Autodesk Inventor part; units mm, degrees
ref_plane "YZ Plane" through (0, 0, 0) normal (1, 0, 0) x (0, 1, 0)
ref_plane "XZ Plane" through (0, 0, 0) normal (0, 1, 0) x (-1, 0, 0)
ref_plane "XY Plane" through (0, 0, 0) normal (0, 0, 1) x (1, 0, 0)
sketch "Sketch6" plane through (0, 0, 0) normal (0, 1, 0) x (-1, 0, 0)
  line L0 (-10, -10) -> (10, -10)
  line L1 (10, -10) -> (10, 10)
  line L2 (10, 10) -> (-10, 10)
  line L3 (-10, 10) -> (-10, -10)
  line L4 (-10, -10) -> (10, 10) construction
  line L5 (10, -10) -> (-10, 10) construction
  point P0 (0, 0)
  dimension "d28" = 20
  dimension "d29" = 20
extrude "Extrusion6" add sketch "Sketch6" along normal blind 1
sketch "Sketch7" plane through (0, 1, 0) normal (0, 1, 0) x (1, 0, 0)
  circle A0 centre (-8.5, -8.5) radius 1
  line L0 (-10, 10) -> (-10, -10)
  line L1 (-10, -10) -> (10, -10)
  point P0 (0, 0)
  dimension "d32" = 2
  dimension "d33" = 0.5
  dimension "d34" = 0.5
extrude "Extrusion7" add sketch "Sketch7" along normal blind 10
sketch "Sketch8" plane through (0, 1, 0) normal (0, 1, 0) x (1, 0, 0)
  circle A0 centre (-8.5, 8.5) radius 1
  line L0 (-10, 10) -> (-10, -10)
  line L1 (10, 10) -> (-10, 10)
  point P0 (0, 0)
  dimension "d37" = 2
  dimension "d38" = 0.5
  dimension "d39" = 0.5
extrude "Extrusion8" add sketch "Sketch8" along normal blind 10
sketch "Sketch9" plane through (0, 1, 0) normal (0, 1, 0) x (1, 0, 0)
  circle A0 centre (8.5, -8.5) radius 1
  line L0 (10, -10) -> (10, 10)
  line L1 (-10, -10) -> (10, -10)
  point P0 (0, 0)
  dimension "d42" = 2
  dimension "d43" = 0.5
  dimension "d44" = 0.5
extrude "Extrusion9" add sketch "Sketch9" along normal blind 10
sketch "Sketch10" plane through (0, 1, 0) normal (0, 1, 0) x (1, 0, 0)
  circle A0 centre (8.5, 8.5) radius 1
  line L0 (10, -10) -> (10, 10)
  line L1 (10, 10) -> (-10, 10)
  point P0 (0, 0)
  dimension "d47" = 2
  dimension "d48" = 0.5
  dimension "d49" = 0.5
extrude "Extrusion10" add sketch "Sketch10" along normal blind 10
sketch "Sketch11" plane through (-8.5, 11, 8.5) normal (0, 1, 0) x (1, 0, 0)
  line L0 (18.75, 18.75) -> (-1.75, 18.75)
  line L1 (-1.75, 18.75) -> (-1.75, -1.75)
  line L2 (-1.75, -1.75) -> (18.75, -1.75)
  line L3 (18.75, -1.75) -> (18.75, 18.75)
  line L4 (18.75, 18.75) -> (-1.75, -1.75) construction
  line L5 (-1.75, 18.75) -> (18.75, -1.75) construction
  point P0 (8.5, 8.5)
  dimension "d52" = 20.5
  dimension "d53" = 20.5
extrude "Extrusion11" add sketch "Sketch11" along normal blind 0.5
sketch "Sketch12" plane through (-8.5, 11.5, 8.5) normal (0, 1, 0) x (1, 0, 0)
  point P0 (8.5, 8.5)
sketch "Sketch13" plane through (-8.5, 11.5, 8.5) normal (0, 1, 0) x (1, 0, 0)
  line L0 (0.75, 0.75) -> (-1.25, 0.75)
  line L1 (-1.25, 0.75) -> (-1.25, -1.25)
  line L2 (-1.25, -1.25) -> (0.75, -1.25)
  line L3 (0.75, -1.25) -> (0.75, 0.75)
  line L4 (0.75, 0.75) -> (-1.25, -1.25) construction
  line L5 (-1.25, 0.75) -> (0.75, -1.25) construction
  line L6 (-1.75, -1.75) -> (18.75, -1.75)
  line L7 (-1.75, 18.75) -> (-1.75, -1.75)
  point P0 (8.5, 8.5)
  point P1 (-0.25, -0.25)
  dimension "d56" = 2
  dimension "d57" = 2
  dimension "d58" = 0.5
  dimension "d59" = 0.5
extrude "Extrusion12" add sketch "Sketch13" along normal blind 10
sketch "Sketch14" plane through (-8.5, 11.5, 8.5) normal (0, 1, 0) x (1, 0, 0)
  line L0 (-1.25, 16.25) -> (0.75, 16.25)
  line L1 (0.75, 16.25) -> (0.75, 18.25)
  line L2 (0.75, 18.25) -> (-1.25, 18.25)
  line L3 (-1.25, 18.25) -> (-1.25, 16.25)
  line L4 (-1.25, 16.25) -> (0.75, 18.25) construction
  line L5 (0.75, 16.25) -> (-1.25, 18.25) construction
  line L6 (-1.75, 18.75) -> (-1.75, -1.75)
  line L7 (18.75, 18.75) -> (-1.75, 18.75)
  point P0 (8.5, 8.5)
  point P1 (-0.25, 17.25)
  dimension "d62" = 2
  dimension "d63" = 2
  dimension "d64" = 0.5
  dimension "d65" = 0.5
extrude "Extrusion13" add sketch "Sketch14" along normal blind 10
sketch "Sketch15" plane through (-8.5, 11.5, 8.5) normal (0, 1, 0) x (1, 0, 0)
  line L0 (18.25, 0.75) -> (16.25, 0.75)
  line L1 (16.25, 0.75) -> (16.25, -1.25)
  line L2 (16.25, -1.25) -> (18.25, -1.25)
  line L3 (18.25, -1.25) -> (18.25, 0.75)
  line L4 (18.25, 0.75) -> (16.25, -1.25) construction
  line L5 (16.25, 0.75) -> (18.25, -1.25) construction
  line L6 (-1.75, -1.75) -> (18.75, -1.75)
  line L7 (18.75, -1.75) -> (18.75, 18.75)
  point P0 (8.5, 8.5)
  point P1 (17.25, -0.25)
  dimension "d68" = 2
  dimension "d69" = 2
  dimension "d70" = 0.5
  dimension "d71" = 0.5
extrude "Extrusion14" add sketch "Sketch15" along normal blind 10
sketch "Sketch16" plane through (-8.5, 11.5, 8.5) normal (0, 1, 0) x (1, 0, 0)
  line L0 (16.25, 16.25) -> (18.25, 16.25)
  line L1 (18.25, 16.25) -> (18.25, 18.25)
  line L2 (18.25, 18.25) -> (16.25, 18.25)
  line L3 (16.25, 18.25) -> (16.25, 16.25)
  line L4 (16.25, 16.25) -> (18.25, 18.25) construction
  line L5 (18.25, 16.25) -> (16.25, 18.25) construction
  line L6 (18.75, -1.75) -> (18.75, 18.75)
  line L7 (18.75, 18.75) -> (-1.75, 18.75)
  point P0 (8.5, 8.5)
  point P1 (17.25, 17.25)
  dimension "d74" = 2
  dimension "d75" = 2
  dimension "d76" = 0.5
  dimension "d77" = 0.5
extrude "Extrusion15" add sketch "Sketch16" along normal blind 10
sketch "Sketch17" plane through (-8.5, 11.5, 8.5) normal (0, 1, 0) x (1, 0, 0)
  line L0 (-1.25, 0.75) -> (0.75, 0.75)
  line L1 (-0.25, 0.75) -> (17.5992, 0.75)
  line L2 (17.5992, 0.75) -> (17.5992, 16.25)
  line L3 (17.5992, 16.25) -> (-0.25, 16.25)
  line L4 (-0.25, 16.25) -> (-0.25, 0.75)
  point P0 (8.5, 8.5)
extrude "Extrusion16" cut sketch "Sketch17" against normal blind 10
sketch "Sketch18" plane through (7.75, 11.5, -9.75) normal (-1, 0, 0) x (0, 0, 1)
  point P0 (9.75, -11.5)
sketch "Sketch19" plane through (7.75, 11.5, -9.75) normal (-1, 0, 0) x (0, 0, 1)
  point P0 (9.75, -11.5)
sketch "Sketch20" plane through (7.75, 11.5, -9.75) normal (-1, 0, 0) x (0, 0, 1)
  point P0 (9.75, -11.5)
sketch "Sketch21" plane through (7.75, 11.5, -9.75) normal (-1, 0, 0) x (0, 0, 1)
  line L0 (2, 8) -> (0, 8)
  line L1 (0, 8) -> (0, 6)
  line L2 (0, 6) -> (2, 6)
  line L3 (2, 6) -> (2, 8)
  line L4 (2, 0) -> (2, 10)
  line L5 (0, 10) -> (2, 10)
  point P0 (9.75, -11.5)
  dimension "d82" = 2
  dimension "d83" = 2
  dimension "d84" = 0
  dimension "d85" = 2
extrude "Extrusion17" add sketch "Sketch21" along normal blind 16
sketch "Sketch22" plane through (7.75, 11.5, 7.75) normal (-1, 0, 0) x (0, 0, 1)
  line L0 (2, 8) -> (0, 8)
  line L1 (0, 8) -> (0, 6)
  line L2 (0, 6) -> (2, 6)
  line L3 (2, 6) -> (2, 8)
  line L4 (2, 0) -> (2, 10)
  line L5 (0, 10) -> (2, 10)
  point P0 (-7.75, -11.5)
  dimension "d88" = 2
  dimension "d89" = 2
  dimension "d90" = 0
  dimension "d91" = 2
extrude "Extrusion18" add sketch "Sketch22" along normal blind 16
sketch "Sketch23" plane through (0, 0, 0) normal (0, -1, 0) x (1, 0, 0)
  circle A0 centre (0, 0) radius 0.5
  dimension "d94" = 1
extrude "Extrusion19" cut sketch "Sketch23" against normal blind 1
properties part number "tABLE" material "Brick, Common, Brown"
Geometry check sheet. Reference: the model listing, model coordinates, mm. A direction names the side the tool comes from. Give positions to 0.01 mm unless a question says otherwise; leave off trailing zeros. Loops run counter-clockwise (first coordinate to the right, second up) from the corner with the lowest first, then second, coordinate; pieces in that order, holes last.
(1) Release check for a two-part mould opening along Z. For faces 1 (the flat face through (-0.1, 0.5, 10)), 2 (the cylindrical face through (-8.63, 5.93, 9.49)), 3 (the flat face through (0.1, 0.5, -10)), 4 (the flat face through (0, 19.5, 9)) record: released by +Z, released by -Z, zero draft, split by the parting line, or undercut.
From the geometry:
face 1: released by +Z
face 2: undercut
face 3: released by -Z
face 4: zero draft
(2) Depth check by flat-ended pin: pin 1 Ø10 at (x, y) = (-4, 4) entering from -Z; pin 2 Ø5 at (x, z) = (-7, -4) entering from -Y; pin 3 Ø1 at (y, z) = (16, -9) entering from -X; pin 4 Ø0.6 at (y, z) = (18.5, -8.5) entering from +X. Enter the tip coordinate at first touch or a pass-through.
From the geometry:
pin 1: stops at z = -10
pin 2: stops at y = 0
pin 3: stops at x = -9.75
pin 4: stops at x = 9.75
(3) Section check B-B on z = -3.5. Record the cut outline in (x, y).
From the geometry:
outline: (-10.25, 11) - (-8.75, 11) - (-8.75, 11.5) - (-10.25, 11.5) - close; (-10, 0) - (10, 0) - (10, 1) - (-10, 1) - close; (9.1, 11) - (10.25, 11) - (10.25, 11.5) - (9.1, 11.5) - close
(4) Section check D-D on x = -6.25. Record the cut outline in (y, z).
From the geometry:
outline: (0, -10) - (1, -10) - (1, 10) - (0, 10) - close; (11, -10.25) - (11.5, -10.25) - (11.5, -7.75) - (11, -7.75) - close; (11, 7.75) - (11.5, 7.75) - (11.5, 10.25) - (11, 10.25) - close; (17.5, -9.75) - (19.5, -9.75) - (19.5, -7.75) - (17.5, -7.75) - close; (17.5, 7.75) - (19.5, 7.75) - (19.5, 9.75) - (17.5, 9.75) - close
(5) Set-up check for faces 5 (the flat face through (-7.75, 20, -9)), 6 (the flat face through (9.75, 16, 9)), 7 (the flat face through (-7.75, 14, -9)), 8 (the flat face through (10, 0.5, 0.1)): record each of +Z, -Z, +X, -X, +Y, -Y from which the full face is reachable in a straight line by a thin tool's end or side.
From the geometry:
face 5: +Z, -Z, +Y
face 6: +Z, -Z, +X, +Y
face 7: +Z, -Z
face 8: +Z, -Z, +X, -Y
(6) Section check C-C on y = 14. Record the cut outline in (x, z), then the cut area to 3 significant figures.
From the geometry:
outline: (-9.75, -9.75) - (-7.75, -9.75) - (-7.75, -7.75) - (-9.75, -7.75) - close; (-9.75, 7.75) - (-7.75, 7.75) - (-7.75, 9.75) - (-9.75, 9.75) - close; (7.75, -9.75) - (9.75, -9.75) - (9.75, -7.75) - (7.75, -7.75) - close; (7.75, 7.75) - (9.75, 7.75) - (9.75, 9.75) - (7.75, 9.75) - close
area: 16.0 mm2
(7) Section check A-A on x = 0. Record the cut outline in (y, z), then the cut area to 3 significant figures.
From the geometry:
outline: (0, -10) - (1, -10) - (1, -0.5) - (0, -0.5) - close; (0, 0.5) - (1, 0.5) - (1, 10) - (0, 10) - close; (11, -10.25) - (11.5, -10.25) - (11.5, -7.75) - (11, -7.75) - close; (11, 7.75) - (11.5, 7.75) - (11.5, 10.25) - (11, 10.25) - close; (17.5, -9.75) - (19.5, -9.75) - (19.5, -7.75) - (17.5, -7.75) - close; (17.5, 7.75) - (19.5, 7.75) - (19.5, 9.75) - (17.5, 9.75) - close
area: 29.5 mm2
(8) Thickness scan on L1, parallel to X at y = 14.25, z = 8.5; L2, parallel to Z at x = 0, y = 0.4; L3, parallel to Y at x = -9.5, z = 4.5. Record the ranges inside material, lowest first.
From the geometry:
L1: x = -9.75 to -7.75, 7.75 to 9.75
L2: z = -10 to -0.5, 0.5 to 10
L3: y = 0 to 1, 11 to 11.5
